from build123d import *

# Parameters (mm, degrees)
F1_DEPTH = 3
F2_W     = 3
F2_H     = 3
F3_DEPTH = 5
F4_R     = 0.65
F5_DEPTH = 7
F6_R     = 1.25
F7_DEPTH = 0.2


with BuildPart() as f1:
    # F0 (on Front) → F1 (new body)
    with BuildSketch(Plane.XZ):
        Polygon((-5, -2.5), (5, -2.5), (5, 2.5), (1.5, 2.5), (-1.5, 2.5), (-5, 2.5), align=None)
    extrude(amount=F1_DEPTH)

    # F2 (on face) → F3 (join)
    with BuildSketch(Plane.XY.offset(2.5)):
        with Locations((0, -1.5)):
            Rectangle(F2_W, F2_H)
    extrude(amount=F3_DEPTH)

    # F4 (on face) → F5 (cut)
    with BuildSketch(Plane.XY.offset(7.5)):
        with Locations((0, -1.5)):
            Circle(F4_R)
    extrude(amount=-F5_DEPTH, mode=Mode.SUBTRACT)

    # F6 (on face) → F7 (cut)
    with BuildSketch(Plane.XY.offset(7.5)):
        with Locations((0, -1.5)):
            Circle(F6_R)
    extrude(amount=-F7_DEPTH, mode=Mode.SUBTRACT)


solid = f1.part
Check sheet for the modelled part. Datum: model origin and axes. Units: mm. A direction names the side the tool comes from. Give positions to 0.01 mm unless a question says otherwise; leave off trailing zeros. Order: outer loops, then holes, each group sorted by start corner. A loop starts at its lowest first (then second) coordinate and runs counter-clockwise, first axis right, second up. Notation, with made-up numbers: (15.5, -3.75) - (54.5, -3.75) arc R23 cw to (54.5, 9.25) - close; hole circle Ø4 at (3.25, -7). An arc over 180 degrees is marked (long way). Answer as CSV lines item,"result".
1. Section check B-B (x = 0). Record the boundary of the cut face in (y, z), then the cut area to 3 significant figures.
Result sheet:
outline,"(-3, -2.5) - (0, -2.5) - (0, 7.5) - (-0.25, 7.5) - (-0.25, 7.3) - (-0.85, 7.3) - (-0.85, 0.5) - (-2.15, 0.5) - (-2.15, 7.3) - (-2.75, 7.3) - (-2.75, 7.5) - (-3, 7.5) - close"
area,"20.7 mm²"
2. Scan lines: probe 1 along Y at (x, z) = (0, 4); probe 2 along Y at (x, z) = (0, 7.4); probe 3 along Z at (x, y) = (-4.25, -0.3). Record each from-to range of solid material in increasing order. Write a range as from..to.
Result sheet:
probe 1,"-3..-2.15, -0.85..0"
probe 2,"-3..-2.75, -0.25..0"
probe 3,"-2.5..2.5"
3. Mould release check, pull along Y, two halves, no side actions. Record for faces 1 (the face through (0, 0, 1)), 2 (the face through (0, -1, -2.5)), 3 (the face through (-0.085, -0.856, 3.948)): released by +Y, released by -Y, zero draft, split by the parting line, or undercut.
Result sheet:
face 1,"released by +Y"
face 2,"zero draft"
face 3,"undercut"
4. Go/stop test with flat-tipped pins: P1, Ø0.8, axis at x = 0.5, y = -2, coming from the +Z side; P2, Ø1.5, axis at x = -3.5, y = -1.5, coming from the +Z side; P3, Ø1.5, axis at y = -0.5, z = 5.5, coming from the -X side. Record where each tip stops, or that it passes through.
Result sheet:
P1,"z = 7.3"
P2,"z = 2.5"
P3,"x = -1.5"
5. Section check D-D (x = 3). Record the boundary of the cut face in (y, z), then the cut area to 3 significant figures.
Result sheet:
outline,"(-3, -2.5) - (0, -2.5) - (0, 2.5) - (-3, 2.5) - close"
area,"15.0 mm²"
6. Section check C-C (y = -1.5). Record the boundary of the cut face in (x, z).
Result sheet:
outline,"(-5, -2.5) - (5, -2.5) - (5, 2.5) - (1.5, 2.5) - (1.5, 7.5) - (1.25, 7.5) - (1.25, 7.3) - (0.65, 7.3) - (0.65, 0.5) - (-0.65, 0.5) - (-0.65, 7.3) - (-1.25, 7.3) - (-1.25, 7.5) - (-1.5, 7.5) - (-1.5, 2.5) - (-5, 2.5) - close"
7. Section check A-A (z = 6). Record the boundary of the cut face in (x, y), then the cut area to 3 significant figures.
Result sheet:
outline,"(-1.5, -3) - (1.5, -3) - (1.5, 0) - (-1.5, 0) - close; hole circle Ø1.3 at (0, -1.5)"
area,"7.67 mm²"
8. Tool access check on faces 4 (the face through (0.8, -1.5, 7.3)), 5 (the face through (-5, -1, 0)), 6 (the face through (1.5, -2, 5)), 7 (the face through (-3, -1, 2.5)). Record the directions out of +Z, -Z, +X, -X, +Y, -Y that give a thin tool (end or side, any length) a straight path to the whole face; none if there is none.
Result sheet:
face 4,"+Z"
face 5,"+Z, -Z, -X, +Y, -Y"
face 6,"+Z, +X, +Y, -Y"
face 7,"+Z, -X, +Y, -Y"
